Work out the finished part from the listing and answer in its coordinate system (mm). A direction names the side the tool comes from. Give positions to 0.01 mm unless a question says otherwise; leave off trailing zeros. Loops run counter-clockwise (first coordinate to the right, second up) from the corner with the lowest first, then second, coordinate; pieces in that order, holes last. Notation, with made-up numbers: M -17.5,-16 L -8.5,-16 A28 ccw -8.5,7 Z; hole C -22,-3 d4. An arc over 180 degrees is marked long. Use a Markdown table: item, result.
```python
from build123d import *

# Parameters (mm, degrees)
BOSS_EXTRUDE1_DEPTH = 4.5
BOSS_EXTRUDE2_DEPTH = 4.5
SKETCH4_R           = 8.1
CUT_EXTRUDE2_DEPTH  = 32.157524023
CUT_EXTRUDE4_REACH  = 33.158
CUT_EXTRUDE5_REACH  = 33.158


with BuildPart() as part:
    # Sketch1 → Boss-Extrude1 (new body)
    with BuildSketch(Plane(origin=(0, 0, 0), x_dir=(1, 0, 0), z_dir=(0, 1, 0))):
        Polygon((-20.25, -13.1232), (20.25, -13.1232), (20.25, -2.125), (1.7907, -2.125), (1.7907, 2.125), (9.398, 2.125), (1.7907, 7.205), (-1.7907, 7.205), (-9.398, 2.125), (-1.7907, 2.125), (-1.7907, -2.125), (-20.25, -2.125), align=None)
    extrude(amount=BOSS_EXTRUDE1_DEPTH)

    # Sketch3 → Boss-Extrude2 (add)
    with BuildSketch(Plane(origin=(0, 4.5, 0), x_dir=(1, 0, 0), z_dir=(0, 1, 0))):
        Polygon((-20.25, -2.125), (-20.25, -13.1232), (20.25, -13.1232), (20.25, -2.125), (1.7907, -2.125), (1.7907, 2.125), (9.398, 2.125), (1.7907, 7.205), (-1.7907, 7.205), (-9.398, 2.125), (-1.7907, 2.125), (-1.7907, -2.125), align=None)
        with BuildLine():
            Line((20.25, -13.1232), (-20.25, -13.1232))
            ThreePointArc((-20.25, -13.1232), (-13.331227209, -22.72714357), (-2.030596131, -19.205654357))
            ThreePointArc((-2.030596131, -19.205654357), (0, -18.191524388), (2.030596131, -19.205654357))
            ThreePointArc((2.030596131, -19.205654357), (13.331227209, -22.72714357), (20.25, -13.1232))
        make_face()
    extrude(amount=-BOSS_EXTRUDE2_DEPTH)

    # Sketch4 → Cut-Extrude2 (cut, through all)
    with BuildSketch(Plane(origin=(0, 4.5, 0), x_dir=(1, 0, 0), z_dir=(0, 1, 0))):
        with Locations(Location((-10.85, -13.1232, 0), (0, 0, 270))):
            Circle(SKETCH4_R)
        with Locations(Location((10.85, -13.1232, 0), (0, 0, 270))):
            Circle(SKETCH4_R)
    extrude(amount=-CUT_EXTRUDE2_DEPTH, mode=Mode.SUBTRACT)

    # Sketch5 → Cut-Extrude4 (cut, up to next)
    with BuildSketch(Plane(origin=(0, 4.5, 0), x_dir=(1, 0, 0), z_dir=(0, 1, 0)), mode=Mode.PRIVATE) as cut_extrude4_sk1:
        with BuildLine():
            Line((7, -5.996665078), (-7, -5.996665078))
            ThreePointArc((-7, -5.996665078), (-3.893168825, -8.974404994), (-2.75, -13.1232))
            Line((-2.75, -13.1232), (2.75, -13.1232))
            ThreePointArc((2.75, -13.1232), (3.893168825, -8.974404994), (7, -5.996665078))
        make_face()
    cut_extrude4_tool1 = extrude(cut_extrude4_sk1.sketch, amount=-CUT_EXTRUDE4_REACH, mode=Mode.PRIVATE) & part.part
    add(cut_extrude4_tool1.solids().sort_by_distance((0, 4.5, 8.978273))[0], mode=Mode.SUBTRACT)

    # Sketch6 → Cut-Extrude5 (cut, up to next)
    with BuildSketch(Plane(origin=(0, 4.5, 0), x_dir=(1, 0, 0), z_dir=(0, 1, 0)), mode=Mode.PRIVATE) as cut_extrude5_sk1:
        with BuildLine():
            Line((-9.2518, -2.125), (-20.25, -2.125))
            Line((-20.25, -2.125), (-20.25, -13.1232))
            ThreePointArc((-20.25, -13.1232), (-17.028701801, -5.346298199), (-9.2518, -2.125))
        make_face()
    cut_extrude5_tool1 = extrude(cut_extrude5_sk1.sketch, amount=-CUT_EXTRUDE5_REACH, mode=Mode.PRIVATE) & part.part
    # Sketch6 → Cut-Extrude5 (cut, up to next)
    with BuildSketch(Plane(origin=(0, 4.5, 0), x_dir=(1, 0, 0), z_dir=(0, 1, 0)), mode=Mode.PRIVATE) as cut_extrude5_sk2:
        with BuildLine():
            Line((20.25, -13.1232), (20.25, -2.125))
            Line((20.25, -2.125), (11.02035, -2.125))
            ThreePointArc((11.02035, -2.125), (17.636860555, -5.94429266), (20.25, -13.1232))
        make_face()
    cut_extrude5_tool2 = extrude(cut_extrude5_sk2.sketch, amount=-CUT_EXTRUDE5_REACH, mode=Mode.PRIVATE) & part.part
    add(cut_extrude5_tool1.solids().sort_by_distance((-17.793355, 4.5, 4.581645))[0], mode=Mode.SUBTRACT)
    add(cut_extrude5_tool2.solids().sort_by_distance((17.919058, 4.5, 4.610875))[0], mode=Mode.SUBTRACT)


solid = part.part
```
(1) A cutting plane is placed at C-C (x = -12). Write down the section's boundary in (y, z), and give its area (3 significant figures).
Entries:
| item | result |
|---|---|
| outline | M 0,2.47 L 4.5,2.47 L 4.5,5.11 L 0,5.11 Z; M 0,21.14 L 4.5,21.14 L 4.5,23.07 L 0,23.07 Z |
| area | 20.5 mm² |
(2) A cutting plane is placed at D-D (z = 4.5). Write down the section's boundary in (x, y), and give its area (3 significant figures).
Entries:
| item | result |
|---|---|
| outline | M -16.08,0 L 16.18,0 L 16.18,4.5 L -16.08,4.5 Z |
| area | 145 mm² |
(3) Given P1, Ø1.3, axis at y = 2, z = 0.5, coming from the -X side; P2, Ø1.5, axis at y = 2.5, z = 15, coming from the +X side; P3, Ø2, axis at x = -7, y = 1.5, coming from the +Z side, each flat-ended and moving along its own axis, determine where each tip first touches the part or whether it passes through.
Entries:
| item | result |
|---|---|
| P1 | stops at x = -1.79 |
| P2 | stops at x = 20.19 |
| P3 | stops at z = 23.02 |
(4) The mould has two halves that part along Z. Classify faces 1 (the flat face through (-5, 2, 2.125)), 2 (the cylindrical face through (-0.03, 2.28, 18.19)), 3 (the flat face through (-5.54, 2.22, -4.7)): released by +Z, released by -Z, zero draft, split by the parting line, or undercut.
Entries:
| item | result |
|---|---|
| face 1 | undercut |
| face 2 | released by +Z |
| face 3 | released by -Z |
(5) Consider probe 1 along Z at (x, y) = (-7, 1.35) (3 decimals); probe 2 along Z at (x, y) = (3.5, 2.9) (3 decimals); probe 3 along X at (y, z) = (1.2, 13). Determine where each line is inside the solid, lowest interval first. Write a range as [from, to].
Entries:
| item | result |
|---|---|
| probe 1 | z = [-3.726, -2.125], [2.125, 5.997], [20.25, 22.754] |
| probe 2 | z = [-6.064, -2.125], [2.125, 5.997], [16.527, 20.78] |
| probe 3 | x = [-20.25, -18.95], [18.95, 20.25] |
(6) Which of the six approach directions +Z, -Z, +X, -X, +Y, -Y give full straight-line access (tool end or side, diameter ignored) to faces 4 (the flat face through (0, 2, 5.997)), 5 (the flat face through (6, 2, -2.125)), 6 (the flat face through (-6, 2, -2.125)), 7 (the flat face through (-0.1, 4.5, 5.7))?
Entries:
| item | result |
|---|---|
| face 4 | +Y, -Y |
| face 5 | +X, +Y, -Y |
| face 6 | -X, +Y, -Y |
| face 7 | +Z, -Z, +X, -X, +Y |
(7) A cutting plane is placed at A-A (x = 0). Write down the section's boundary in (y, z) (3 decimals), and give its area (3 significant figures).
Entries:
| item | result |
|---|---|
| outline | M 0,-7.205 L 4.5,-7.205 L 4.5,5.997 L 0,5.997 Z; M 0,13.123 L 4.5,13.123 L 4.5,18.192 L 0,18.192 Z |
| area | 82.2 mm² |
(8) A cutting plane is placed at B-B (y = 3.85). Write down the section's boundary in (x, z) (3 decimals).
Entries:
| item | result |
|---|---|
| outline | M -20.25,13.123 A10.998 ccw -9.252,2.125 L -1.791,2.125 L -1.791,-2.125 L -9.398,-2.125 L -1.791,-7.205 L 1.791,-7.205 L 9.398,-2.125 L 1.791,-2.125 L 1.791,2.125 L 11.02,2.125 A11.168 ccw 20.25,13.123 A10.125 ccw 2.031,19.206 A2.54 cw -2.031,19.206 A10.125 ccw Z; hole M -7,5.997 L 7,5.997 A8.1 ccw long 2.75,13.123 L -2.75,13.123 A8.1 ccw long Z |
